```python
from build123d import *
from build123d.topology import SkipClean

# Parameters (mm, degrees)
CUT_EXTRUDE3_DEPTH = 17.226666346
CUT_EXTRUDE4_DEPTH = 10.882576389
CUT_EXTRUDE5_DEPTH = 1
CUT_EXTRUDE5_DRAFT = -25
CUT_EXTRUDE7_START = -7
CUT_EXTRUDE7_DEPTH = 5
CUT_EXTRUDE8_START = -1
CUT_EXTRUDE8_DEPTH = 6


with BuildPart() as part:
    # Sketch2 → Revolve1 (revolve)
    with BuildSketch(Plane.XY, mode=Mode.PRIVATE) as revolve1_sk:
        with BuildLine():
            Line((-6.63150289, 0), (-6.63150289, 1.625))
            Line((-6.63150289, 1.625), (1.26849711, 1.625))
            ThreePointArc((1.26849711, 1.625), (2.178863013, 2.343741755), (3.310095748, 2.6))
            Line((3.310095748, 2.6), (6.510095748, 2.50867829))
            ThreePointArc((6.510095748, 2.50867829), (8.318770507, 1.760874291), (9.17307545, 0))
            Line((9.17307545, 0), (-6.63150289, 0))
        make_face()
    revolve(revolve1_sk.sketch.rotate(Axis((-13.79438497, 0, 0), (1, 0, 0)), 90), axis=Axis((-13.79438497, 0, 0), (1, 0, 0)))

    # Sketch8 → Cut-Extrude3 (cut, through all)
    with SkipClean():  # the faces are left unmerged after this step: merging them gives an invalid solid
        with BuildSketch(Plane.ZY.offset(6.63150289)):
            with BuildLine():
                Line((0, -1.625), (0, -2.6))
                ThreePointArc((0, -2.6), (-2.6, 0), (0, 2.6))
                Line((0, 2.6), (0, 1.625))
                ThreePointArc((0, 1.625), (-1.625, 0), (0, -1.625))
            make_face()
        extrude(amount=-CUT_EXTRUDE3_DEPTH, mode=Mode.SUBTRACT)

    # Sketch9 → Cut-Extrude4 (cut, through all)
    with SkipClean():  # the faces are left unmerged after this step: merging them gives an invalid solid
        with BuildSketch(Plane(origin=(0, 0, 0), x_dir=(-1, 0, 0), z_dir=(0, 0, -1))):
            with BuildLine():
                Line((-1.26849711, 1.625), (-1.26849711, -1.625))
                Line((-1.26849711, -1.625), (-2.014389305, -1.625))
                ThreePointArc((-2.014389305, -1.625), (-4.93682915, -1.903834504), (-7.859268995, -1.625))
                Line((-7.859268995, -1.625), (-8.453314596, -1.625))
                ThreePointArc((-8.453314596, -1.625), (-9.31617507, 0), (-8.453314596, 1.625))
                Line((-8.453314596, 1.625), (-7.859268995, 1.625))
                ThreePointArc((-7.859268995, 1.625), (-4.926626022, 1.952572443), (-1.993983049, 1.625))
                Line((-1.993983049, 1.625), (-1.26849711, 1.625))
            make_face()
        extrude(amount=CUT_EXTRUDE4_DEPTH, mode=Mode.SUBTRACT)


with BuildPart() as cut_extrude5_tool:
    # Sketch10 → Cut-Extrude5 (with draft: the straight prism first)
    with BuildSketch(Plane(origin=(0, 0, 0), x_dir=(-1, 0, 0), z_dir=(0, 0, -1))):
        with BuildLine():
            ThreePointArc((-6.754616043, 1.962865993), (-8.41489063, 0), (-6.754616043, -1.962865993))
            Line((-6.754616043, -1.962865993), (-2.943623614, -1.962865993))
            ThreePointArc((-2.943623614, -1.962865993), (-1.898821514, 0), (-2.943623614, 1.962865993))
            Line((-2.943623614, 1.962865993), (-6.754616043, 1.962865993))
        make_face()
    extrude(amount=-CUT_EXTRUDE5_DEPTH)
    # Cut-Extrude5: the draft: its side faces are tilted about the plane it starts from
    cut_extrude5_sides = [cut_extrude5_tool.faces().sort_by_distance(p)[0] for p in [
        (4.849119829, -1.962865993, 0.5),
        (1.898821514, 0, 0.5),
        (4.849119829, 1.962865993, 0.5),
        (8.41489063, 0, 0.5),
    ]]
    draft(cut_extrude5_sides, Plane(origin=(0, 0, 0), x_dir=(-1, 0, 0), z_dir=(0, 0, -1)), CUT_EXTRUDE5_DRAFT)


with BuildPart() as part_1:
    add(part.part)

    # Cut-Extrude5: cut by cut_extrude5_tool
    add(cut_extrude5_tool.part, mode=Mode.SUBTRACT)

    # Sketch13 → Cut-Extrude7 (cut)
    with BuildSketch(Plane.ZY.offset(6.63150289).offset(CUT_EXTRUDE7_START)):
        with BuildLine():
            Line((1.270607087, -1.013006727), (1.270607087, 1.013006727))
            ThreePointArc((1.270607087, 1.013006727), (1.625, 0), (1.270607087, -1.013006727))
        make_face()
    extrude(amount=CUT_EXTRUDE7_DEPTH, mode=Mode.SUBTRACT)

    # Sketch14 → Cut-Extrude8 (cut)
    with BuildSketch(Plane(origin=(1.26849711, 0, 0), x_dir=(0, 0, -1), z_dir=(1, 0, 0)).offset(CUT_EXTRUDE8_START)):
        with BuildLine():
            Line((1.153512248, 1.144567383), (1.153512248, -1.144567383))
            ThreePointArc((1.153512248, -1.144567383), (1.625, 0), (1.153512248, 1.144567383))
        make_face()
    extrude(amount=-CUT_EXTRUDE8_DEPTH, mode=Mode.SUBTRACT)


solid = part_1.part
```
Geometry check sheet. Reference: the model listing, model coordinates, mm. A direction names the side the tool comes from. Coordinates: 2 decimals unless noted, no trailing zeros. Order: outer loops, then holes, each group sorted by start corner. A loop starts at its lowest first (then second) coordinate and runs counter-clockwise, first axis right, second up.
Q1. Sectioned sample at B-B on x = -2. Record the cut outline in (y, z) (3 decimals), and give its area (3 significant figures).
Reply:
outline: (-1.145, -1.154) - (1.145, -1.154) arc R1.625 ccw to (1.013, 1.271) - (-1.013, 1.271) arc R1.625 ccw to start
area: 7.06 mm2
Q2. Sectioned sample at A-A on z = -1. Record the cut outline in (x, y).
Reply:
outline: (-6.63, -1.28) - (1.27, -1.28) - (1.27, 1.28) - (-6.63, 1.28) - close
Q3. Thickness scan on probe 1 along X at (y, z) = (0.9, -1.2); probe 2 along Y at (x, z) = (-5, 1.15); probe 3 along Z at (x, y) = (-3, -0.15). Record the ranges inside material, lowest first.
Reply:
probe 1: x = -6.63 to -5.73, 0.27 to 1.27
probe 2: y = -1.15 to 1.15
probe 3: z = -1.15 to 1.27
Q4. Tool access check on faces 4 (the face through (-3, 0, -1.154)), 5 (the face through (4.876, -1.733, 0.493)), 6 (the face through (4.932, 0.056, 2.553)), 7 (the face through (-2, 0, 1.271)). Record the directions out of +Z, -Z, +X, -X, +Y, -Y that give a thin tool (end or side, any length) a straight path to the whole face; none if there is none.
Reply:
face 4: -Z, +Y, -Y
face 5: -Z
face 6: +Z, +X
face 7: +Z, +Y, -Y
Q5. Draft check along Y on faces 1 (the face through (5.2, 2.13, 0)), 2 (the face through (-2.63, 1.44, 0.75)), 3 (the face through (4.822, 1.733, 0.493)). Enter one of: released by +Y, released by -Y, zero draft, split by the parting line, or undercut.
Reply:
face 1: zero draft
face 2: split by the parting line
face 3: undercut
Q6. Depth check by flat-ended pin: pin 1 Ø2 at (x, y) = (-1, -0.5) entering from +Z; pin 2 Ø0.5 at (y, z) = (-0.5, -1.5) entering from +X; pin 3 Ø0.7 at (x, y) = (-1.5, 0) entering from -Z. Enter the tip coordinate at first touch or a pass-through.
Reply:
pin 1: stops at z = 1.27
pin 2: stops at x = 1.27
pin 3: stops at z = -1.15
